from build123d import *

# Parameters (mm, degrees)
PAD_DEPTH           = 20
SKETCH001_R         = 5.25
POCKET_DEPTH        = 15
HOLE_D              = 5.5
HOLE_CSINK_D        = 10
HOLE_CSINK_ANGLE    = 90
POCKET001_DEPTH     = 3
FILLET_R            = 4
HOLE001_D           = 5.5
HOLE001_DEPTH       = 25
HOLE001_CSINK_D     = 10
HOLE001_CSINK_ANGLE = 90
POCKET002_DEPTH     = 3


with BuildPart() as part:
    # Sketch → Pad (new body)
    with BuildSketch(Plane.XY):
        with BuildLine():
            Line((-30, 10), (0, 10))
            Line((0, 10), (0, -10))
            Line((0, -10), (-30, -10))
            ThreePointArc((-30, 10), (-40, 0), (-30, -10))
        make_face()
    extrude(amount=PAD_DEPTH)

    # Sketch001 (on Face2 of Pad) → Pocket (cut)
    with BuildSketch(Plane.YZ):
        with Locations((0, 10)):
            Circle(SKETCH001_R)
    extrude(amount=-POCKET_DEPTH, mode=Mode.SUBTRACT)

    # Hole (through all)
    with Locations(Plane.XZ.offset(10)):
        with Locations((-8.827239, 10)):
            CounterSinkHole(HOLE_D / 2, HOLE_CSINK_D / 2, counter_sink_angle=HOLE_CSINK_ANGLE)

    # Sketch004 (on Face1 of Hole) → Pocket001 (cut)
    with BuildSketch(Plane(origin=(0, 10, 0), x_dir=(-1, 0, 0), z_dir=(0, 1, 0))):
        Polygon((11.165508, 5.95), (13.503776, 10), (11.165508, 14.05), (6.48897, 14.05), (4.150702, 10), (6.48897, 5.95), align=None)
    extrude(amount=-POCKET001_DEPTH, mode=Mode.SUBTRACT)

    # Fillet
    fillet_edges = [part.edges().sort_by_distance(p)[0] for p in [
        (-15, -10, 0),
        (-40, 0, 0),
        (-15, 10, 0),
        (-40, 0, 20),
        (-15, 10, 20),
    ]]
    fillet(fillet_edges, radius=FILLET_R)

    # Hole001
    with Locations(Plane(origin=(0, 0, 0), x_dir=(1, 0, 0), z_dir=(0, 0, -1))):
        with Locations((-30, 0)):
            CounterSinkHole(HOLE001_D / 2, HOLE001_CSINK_D / 2, depth=HOLE001_DEPTH, counter_sink_angle=HOLE001_CSINK_ANGLE)

    # Sketch006 (on Face16 of Hole001) → Pocket002 (cut)
    with BuildSketch(Plane.XY.offset(20)):
        Polygon((-27.661731, -4.05), (-25.323463, 0), (-27.661731, 4.05), (-32.338269, 4.05), (-34.676537, 0), (-32.338269, -4.05), align=None)
    extrude(amount=-POCKET002_DEPTH, mode=Mode.SUBTRACT)


solid = part.part
Can you work these out from the model? Positions are in its coordinate system, mm. A direction names the side the tool comes from. Round coordinates to 2 decimals unless told otherwise and drop trailing zeros. Write each loop counter-clockwise with the first axis right and the second up, starting at its lowest first coordinate (ties: lowest second). Pieces come first, ordered by that corner, then holes. Notation, with made-up numbers: M 24.25,22 L 57.25,22 A30 cw 57.25,60 Z; hole C -28,8 d8. An arc over 180 degrees is marked long. Use a Markdown table: item, result.
Item 1: I want a section at B-B (z = 12). State how many separate pieces and enclosed holes the cut face has, and give its area (3 significant figures).
Found:
| item | result |
|---|---|
| separate pieces | 3 |
| enclosed holes | 1 |
| area | 533 mm2 |
Item 2: I want a section at A-A (z = 3.5). List the corners of the cut face in (x, y) for me, and give its area (3 significant figures).
Found:
| item | result |
|---|---|
| outline | M -30,-9.97 L 0,-9.97 L 0,9.97 L -30,9.97 A9.97 ccw Z; hole C -30,0 d5.5 |
| area | 730 mm2 |
Item 3: We'd pull the mould along Y, two halves only. Please class faces 1 (the face through (-9, 7, 13)), 2 (the face through (-5.336, 8.521, 12.053)), 3 (the face through (-30, 3, 17)), 4 (the face through (-18, -10, 10)): released by +Y, released by -Y, zero draft, split by the parting line, or undercut.
Found:
| item | result |
|---|---|
| face 1 | released by +Y |
| face 2 | zero draft |
| face 3 | undercut |
| face 4 | released by -Y |
Item 4: Which directions (+Z, -Z, +X, -X, +Y, -Y) give clear straight access to the entire face, cutting with the end or side of a thin tool? Please do faces 5 (the face through (-26.509, -2.053, 18.521)), 6 (the face through (-12.32, 8.52, 7.95)), 7 (the face through (-14, 0, 20)), 8 (the face through (-15, 0, 10)), 9 (the face through (-15.21, 8.859, 18.797)).
Found:
| item | result |
|---|---|
| face 5 | +Z |
| face 6 | +Y |
| face 7 | +Z, +X, -X, +Y, -Y |
| face 8 | +X |
| face 9 | +Z, +X, -X, +Y |
Item 5: If I drill on line 1 along Z through (x, y) = (-8.75, 0); line 2 along X through (y, z) = (8.75, 6); line 3 along Z through (x, y) = (-13.5, -3), over which ranges is the centre line in solid material (lowest first)? Write a range as [from, to].
Found:
| item | result |
|---|---|
| line 1 | z = [0, 4.75], [15.25, 20] |
| line 2 | x = [-34.84, -11.19], [-6.46, 0] |
| line 3 | z = [0, 5.69], [14.31, 20] |
Item 6: For pin 1 Ø2 at (y, z) = (4.5, 13) entering from -X; pin 2 Ø0.9 at (x, y) = (-8, 8) entering from -Z; pin 3 Ø2.5 at (x, z) = (-31, 19) entering from -Y; pin 4 Ø5 at (x, y) = (-30, 0) entering from -Z, each with a flat end and sliding along its axis, tell me the tip position at first contact or that it passes through.
Found:
| item | result |
|---|---|
| pin 1 | stops at x = -39.37 |
| pin 2 | stops at z = 0.31 |
| pin 3 | stops at y = -9.56 |
| pin 4 | passes through |
